from build123d import *

# Parameters (mm, degrees)
F1_DEPTH = 5


with BuildPart() as f1:
    # F0 (on Right) → F1 (new body)
    with BuildSketch(Plane.YZ):
        Polygon((37.5, 58), (37.5, 65), (9, 65), (9, 70), (-9, 70), (-9, 65), (-37.5, 65), (-37.5, 58), (-42.5, 58), (-42.5, 40), (-37.5, 40), (-37.5, -40), (-42.5, -40), (-42.5, -58), (-37.5, -58), (-37.5, -65), (-9, -65), (-9, -70), (9, -70), (9, -65), (37.5, -65), (37.5, -58), (42.5, -58), (42.5, -40), (37.5, -40), (37.5, 40), (42.5, 40), (42.5, 58), align=None)
    extrude(amount=F1_DEPTH)


solid = f1.part
Here's how the part is built. I have some questions about the finished solid (model axes, mm). A direction names the side the tool comes from. Round coordinates to 2 decimals unless told otherwise and drop trailing zeros. Loops run counter-clockwise (first coordinate to the right, second up) from the corner with the lowest first, then second, coordinate; pieces in that order, holes last. Notation, with made-up numbers: (66, 83) -> (118, 83) arc R30 ccw to (118, 119) -> close; hole circle Ø8 at (-17.75, 13.25). An arc over 180 degrees is marked (long way). Write each question's results on one line, items separated by ' | '.
(1) If we section it at B-B, the plane z = -21: List the corners of the cut face in (x, y) for me.
Worked answers:
outline: (0, -37.5) -> (5, -37.5) -> (5, 37.5) -> (0, 37.5) -> close
(2) For P1, Ø2.5, axis at x = 3.5, y = -39, coming from the +Z side; P2, Ø2.5, axis at x = 1.5, y = -39.5, coming from the -Z side; P3, Ø2, axis at y = -4.5, z = -53.5, coming from the -X side; P4, Ø1, axis at x = 1.5, z = 11, coming from the +Y side, each with a flat end and sliding along its axis, tell me the tip position at first contact or that it passes through.
Worked answers:
P1: z = 58 | P2: z = -58 | P3: x = 0 | P4: y = 37.5
(3) If we section it at A-A, the plane x = 2.8: List the corners of the cut face in (y, z) for me, then the cut area to 3 significant figures.
Worked answers:
outline: (-42.5, -58) -> (-37.5, -58) -> (-37.5, -65) -> (-9, -65) -> (-9, -70) -> (9, -70) -> (9, -65) -> (37.5, -65) -> (37.5, -58) -> (42.5, -58) -> (42.5, -40) -> (37.5, -40) -> (37.5, 40) -> (42.5, 40) -> (42.5, 58) -> (37.5, 58) -> (37.5, 65) -> (9, 65) -> (9, 70) -> (-9, 70) -> (-9, 65) -> (-37.5, 65) -> (-37.5, 58) -> (-42.5, 58) -> (-42.5, 40) -> (-37.5, 40) -> (-37.5, -40) -> (-42.5, -40) -> close | area: 10,300 mm2
(4) We'd pull the mould along Z, two halves only. Please class faces 4 (the face through (2, 37.5, -62)), 5 (the face through (2, 40, -40)), 6 (the face through (2, -40, 58)): released by +Z, released by -Z, zero draft, split by the parting line, or undercut.
Worked answers:
face 4: zero draft | face 5: undercut | face 6: released by +Z
(5) If we section it at C-C, the plane y = -19.5: List the corners of the cut face in (x, z) for me, then the cut area to 3 significant figures.
Worked answers:
outline: (0, -65) -> (5, -65) -> (5, 65) -> (0, 65) -> close | area: 650 mm2
(6) For faces 1 (the face through (2, 23, 65)), 2 (the face through (2, -9, 68)), 3 (the face through (2, -37.5, -61)), which set-ups out of +Z, -Z, +X, -X, +Y, -Y let a thin tool reach every point of the face, with its end or its side?
Worked answers:
face 1: +Z, +X, -X, +Y | face 2: +Z, +X, -X, -Y | face 3: -Z, +X, -X, -Y
(7) If I drill on L1, parallel to Z at x = 2.3, y = -27; L2, parallel to Y at x = 0.95, z = 19, over which ranges is the centre line in solid material (lowest first)?
Worked answers:
L1: -65 to 65 | L2: -37.5 to 37.5
